Verification items for the finished model (mm, model axes). A direction names the side the tool comes from. Give positions to 0.01 mm unless a question says otherwise; leave off trailing zeros. Loops run counter-clockwise (first coordinate to the right, second up) from the corner with the lowest first, then second, coordinate; pieces in that order, holes last. Notation, with made-up numbers: M -24.5,33 L 19.5,33 A35 cw 19.5,67 Z; hole C 6.5,74 d11. An arc over 180 degrees is marked long. Answer in a Markdown table with one row per item.
```python
from build123d import *

# Parameters (mm, degrees)
SKETCH1_W                = 200
SKETCH1_H                = 200
BOSS_EXTRUDE1_DEPTH      = 3
SKETCH2_R                = 13
SKETCH2_R_2              = 35.7386452
SKETCH2_R_3              = 0.8
CUT_EXTRUDE1_DEPTH       = 283.85862193
M3_CLEARANCE_HOLE1_D     = 3.4
SKETCH5_R                = 13
CUT_EXTRUDE2_DEPTH       = 1
SKETCH6_W                = 50
SKETCH6_H                = 200
SKETCH6_W_2              = 100
BOSS_EXTRUDE2_DEPTH      = 3
M4_CLEARANCE_HOLE1_D     = 4.5
M4_CLEARANCE_HOLE1_DEPTH = 7
M4_CLEARANCE_HOLE1_TIP   = 1.351936393
M4_CLEARANCE_HOLE2_D     = 4.5
M4_CLEARANCE_HOLE2_DEPTH = 7
M4_CLEARANCE_HOLE2_TIP   = 1.351936393


with BuildPart() as part:
    # Sketch1 → Boss-Extrude1 (new body)
    with BuildSketch(Plane(origin=(0, 0, 0), x_dir=(1, 0, 0), z_dir=(0, 1, 0))):
        with Locations((100, 100)):
            Rectangle(SKETCH1_W, SKETCH1_H)
    extrude(amount=BOSS_EXTRUDE1_DEPTH)

    # Sketch2 → Cut-Extrude1 (cut, through all)
    with BuildSketch(Plane(origin=(0, 3, 0), x_dir=(1, 0, 0), z_dir=(0, 1, 0))):
        with Locations(Location((50.001332131, 59.483836796, 0), (0, 0, 270))):
            Circle(SKETCH2_R)
        with Locations(Location((150, 60, 0), (0, 0, 270))):
            Circle(SKETCH2_R)
        with Locations(Location((150, 160, 0), (0, 0, 270))):
            Circle(SKETCH2_R_2)
        with Locations(Location((46.591949224, 172.263872743, 0), (0, 0, 270))):
            Circle(SKETCH2_R_3)
        with Locations(Location((64.370811118, 171.396653192, 0), (0, 0, 90))):
            Circle(SKETCH2_R_3)
        with BuildLine():
            Line((73.052642061, 49.602687546), (72.949409421, 69.60242112))
            ThreePointArc((72.949409421, 69.60242112), (74.939059514, 71.612717742), (76.949356135, 69.623067648))
            Line((76.949356135, 69.623067648), (77.052588776, 49.623334074))
            ThreePointArc((77.052588776, 49.623334074), (75.062938683, 47.613037453), (73.052642061, 49.602687546))
        make_face()
        with BuildLine():
            Line((62.029703942, 166.504903281), (62.354703913, 173.16772538))
            ThreePointArc((62.354703913, 173.16772538), (55.639330891, 175.068409569), (48.770854376, 173.830320093))
            Line((48.770854376, 173.830320093), (48.445854405, 167.167497995))
            ThreePointArc((48.445854405, 167.167497995), (54.380843153, 149.268161339), (62.029703942, 166.504903281))
        make_face()
        with BuildLine():
            Line((62.877372778, 118.201780064), (42.901123459, 119.176184054))
            ThreePointArc((42.901123459, 119.176184054), (41.000938926, 121.271249385), (43.096004257, 123.171433918))
            Line((43.096004257, 123.171433918), (63.072253576, 122.197029928))
            ThreePointArc((63.072253576, 122.197029928), (64.972438109, 120.101964597), (62.877372778, 118.201780064))
        make_face()
    extrude(amount=-CUT_EXTRUDE1_DEPTH, mode=Mode.SUBTRACT)

    # M3 Clearance Hole1 (through all)
    with Locations(Plane(origin=(0, 3, 0), x_dir=(1, 0, 0), z_dir=(0, 1, 0))):
        with Locations((132.5, 60), (150, 77.5), (150, 42.5), (167.5, 60), (50.001332131, 76.983836796), (50.001332131, 41.983836796), (67.501332131, 59.483836796), (32.501332131, 59.483836796)):
            Hole(M3_CLEARANCE_HOLE1_D / 2)

    # Sketch5 → Cut-Extrude2 (cut)
    with BuildSketch(Plane(origin=(0, 3, 0), x_dir=(1, 0, 0), z_dir=(0, 1, 0))):
        with Locations((54.873352081, 159.365083393)):
            Circle(SKETCH5_R)
    extrude(amount=-CUT_EXTRUDE2_DEPTH, mode=Mode.SUBTRACT)

    # Sketch6 → Boss-Extrude2 (add)
    with BuildSketch(Plane(origin=(0, 3, 0), x_dir=(1, 0, 0), z_dir=(0, 1, 0))):
        with Locations((-25, 100)):
            Rectangle(SKETCH6_W, SKETCH6_H)
        with Locations((250, 100)):
            Rectangle(SKETCH6_W_2, SKETCH6_H)
    extrude(amount=-BOSS_EXTRUDE2_DEPTH)

    # M4 Clearance Hole1
    with Locations(Plane(origin=(0, 3, 0), x_dir=(1, 0, 0), z_dir=(0, 1, 0))):
        with Locations((100, 170), (250, 170), (250, 70)):
            Hole(M4_CLEARANCE_HOLE1_D / 2, depth=M4_CLEARANCE_HOLE1_DEPTH)
            with Locations((0, 0, -(M4_CLEARANCE_HOLE1_DEPTH + M4_CLEARANCE_HOLE1_TIP / 2))):  # 118° drill point
                Cone(0, M4_CLEARANCE_HOLE1_D / 2, M4_CLEARANCE_HOLE1_TIP, mode=Mode.SUBTRACT)

    # M4 Clearance Hole2
    with Locations(Plane(origin=(0, 3, 0), x_dir=(1, 0, 0), z_dir=(0, 1, 0))):
        with Locations((-20, 30), (270, 30), (-20, 170), (270, 170), (120, 110), (120, 30)):
            Hole(M4_CLEARANCE_HOLE2_D / 2, depth=M4_CLEARANCE_HOLE2_DEPTH)
            with Locations((0, 0, -(M4_CLEARANCE_HOLE2_DEPTH + M4_CLEARANCE_HOLE2_TIP / 2))):  # 118° drill point
                Cone(0, M4_CLEARANCE_HOLE2_D / 2, M4_CLEARANCE_HOLE2_TIP, mode=Mode.SUBTRACT)


solid = part.part
```
Item 1: Sectioned sample at A-A (x = 176). Record the cut outline in (y, z), and give its area (3 significant figures).
Reported:
| item | result |
|---|---|
| outline | M 0,-200 L 3,-200 L 3,-184.52 L 0,-184.52 Z; M 0,-135.48 L 3,-135.48 L 3,0 L 0,0 Z |
| area | 453 mm^2 |
Item 2: Scan lines: L1, parallel to X at y = 2.55, z = -150; L2, parallel to X at y = 0.85, z = -70; L3, parallel to Z at x = 50.5, y = 0.45. Record each from-to range of solid material in increasing order. Write a range as [from, to].
Reported:
| item | result |
|---|---|
| L1 | x = [-50, 45.86], [63.89, 115.69], [184.31, 300] |
| L2 | x = [-50, 42.36], [57.64, 72.99], [76.91, 141.69], [158.31, 247.75], [252.25, 300] |
| L3 | z = [-200, -174.45], [-150.25, -122.81], [-118.81, -78.61], [-75.36, -72.47], [-46.49, -43.61], [-40.36, 0] |
Item 3: Release check for a two-part mould opening along X. For faces 3 (the flat face through (123, 0, -101)), 4 (the cylindrical face through (137.31, 1.52, -62.82)) record: released by +X, released by -X, zero draft, split by the parting line, or undercut.
Reported:
| item | result |
|---|---|
| face 3 | zero draft |
| face 4 | undercut |
Item 4: Sectioned sample at B-B (y = 1.1). State how many separate pieces and enclosed holes the cut face has, and give its area (3 significant figures).
Reported:
| item | result |
|---|---|
| separate pieces | 1 |
| enclosed holes | 25 |
| area | 64,100 mm^2 |
Item 5: Tool access check on faces 1 (the cylindrical face through (160.7, 1.5, -125.9)), 2 (the flat face through (50, 2, -150)). Record the directions out of +Z, -Z, +X, -X, +Y, -Y that give a thin tool (end or side, any length) a straight path to the whole face; none if there is none.
Reported:
| item | result |
|---|---|
| face 1 | +Y, -Y |
| face 2 | +Y |
